```python
from build123d import *

# Parameters (mm, degrees)
PAD_DEPTH    = 1
SKETCH001_R  = 2.8
PAD001_DEPTH = 2.5
PAD002_DEPTH = 2
BOX_W        = 14
BOX_H        = 15.5
BOX_DEPTH    = 2


with BuildPart() as pad002:
    # Sketch → Pad (new body)
    with BuildSketch(Plane.XZ):
        with BuildLine():
            Line((-8.098338, 6.85), (11.901662, 6.85))
            Line((11.901662, 6.85), (11.901662, -6.85))
            Line((11.901662, -6.85), (-8.098338, -6.85))
            ThreePointArc((-8.098338, 6.85), (-14.94833, 0), (-8.098338, -6.85))
        make_face()
    extrude(amount=PAD_DEPTH)

    # Sketch001 → Pad001 (new body)
    with BuildSketch(Plane.XZ.offset(1)):
        with Locations((-8.09833, 0)):
            Circle(SKETCH001_R)
    extrude(amount=PAD001_DEPTH)

    # Sketch002 → Pad002 (new body)
    with BuildSketch(Plane.XZ.offset(1)):
        with BuildLine():
            Line((-4.392837, 6.85), (11.900914, 6.85))
            Line((11.900914, 6.85), (11.900914, -6.85))
            Line((11.900914, -6.85), (-4.392837, -6.85))
            ThreePointArc((-4.392837, -6.85), (-0.92548, 0), (-4.392837, 6.85))
        make_face()
    extrude(amount=PAD002_DEPTH)


with BuildPart() as part_mirroring:
    # Part__Mirroring: instance of Pad002
    add(pad002.part.mirror(Plane(origin=(0, 4.75, 0), x_dir=(1, 0, 0), z_dir=(0, 1, 0))))


with BuildPart() as fusion:
    # Box → Box (new body)
    with BuildSketch(Plane(origin=(-2.1, -3, -6.85), x_dir=(1, 0, 0), z_dir=(0, 0, 1))):
        with Locations((7, 7.75)):
            Rectangle(BOX_W, BOX_H)
    extrude(amount=BOX_DEPTH)

    # Fusion: union Pad002, Part__Mirroring
    add(pad002.part)
    add(part_mirroring.part)


solid = fusion.part
```
The listing builds one solid part. Answer for the finished solid, in the listing's coordinates (mm). A direction names the side the tool comes from. Give positions to 0.01 mm unless a question says otherwise; leave off trailing zeros. Order: outer loops, then holes, each group sorted by start corner. A loop starts at its lowest first (then second) coordinate and runs counter-clockwise, first axis right, second up. Notation, with made-up numbers: (43, 30.5) - (100, 30.5) arc R29 cw to (100, 57.5) - close; hole circle Ø2 at (80, -37). An arc over 180 degrees is marked (long way). Answer in a Markdown table with one row per item. Add a question column.
Q1. Find the intervals of material crossed by line 1 along Y through (x, z) = (5, -1.5); line 2 along Y through (x, z) = (-6.75, -4.5); line 3 along Z through (x, y) = (4.75, 8), in increasing order. Write a range as [from, to].
Q2. The part is cut by section C-C (x = -0.5). Determine the outline of the cut face in (y, z).
Q3. Which of the six approach directions +Z, -Z, +X, -X, +Y, -Y give full straight-line access (tool end or side, diameter ignored) to faces 1 (the flat face through (-8, 10.5, 3)), 2 (the flat face through (-2.1, 5, -6)), 3 (the cylindrical face through (-0.926, -1.986, -0.112)), 4 (the flat face through (5, 5, -4.85))?
Q4. The part is cut by section A-A (y = 11.25). Determine the outline of the cut face in (x, z), then the cut area to 3 significant figures.
Q5. For a pull along Z with two mould halves and no side action, classify faces 5 (the cylindrical face through (-0.926, 11.486, -0.112)), 6 (the cylindrical face through (-5.428, -2.232, 0.841)), 7 (the flat face through (-8, -1, 3)), 8 (the flat face through (4, 11, 6.85)) as released by +Z, released by -Z, zero draft, split by the parting line, or undercut.
Q6. Given P1, Ø7, axis at x = 3.5, z = -2.5, coming from the +Y side; P2, Ø7, axis at x = 7, z = -1, coming from the -Y side; P3, Ø1, axis at x = -11.5, z = 3.5, coming from the +Y side, each flat-ended and moving along its own axis, determine where each tip first touches the part or whether it passes through.
Determined:
| question | item | result |
|---|---|---|
| 1 | line 1 | y = [-3, 0], [9.5, 12.5] |
| 1 | line 2 | y = [-1, 0], [9.5, 10.5] |
| 1 | line 3 | z = [-6.85, -4.85] |
| 2 | outline | (-3, -6.85) - (12.5, -6.85) - (12.5, 6.85) - (9.5, 6.85) - (9.5, -4.85) - (0, -4.85) - (0, 6.85) - (-3, 6.85) - close |
| 3 | face 1 | +Y |
| 3 | face 2 | +Z, -Z, -X |
| 3 | face 3 | -Y |
| 3 | face 4 | +Z, +X, -X |
| 4 | outline | circle Ø5.6 at (-8.1, 0); (-4.39, -6.85) - (11.9, -6.85) - (11.9, 6.85) - (-4.39, 6.85) arc R8.5 cw to start |
| 4 | area | 215 mm² |
| 5 | face 5 | undercut |
| 5 | face 6 | split by the parting line |
| 5 | face 7 | undercut |
| 5 | face 8 | released by +Z |
| 6 | P1 | stops at y = 12.5 |
| 6 | P2 | stops at y = -3 |
| 6 | P3 | stops at y = 10.5 |
